Drawing for the job (mm, zero at the part's lowest x, y, z). A direction names the side the tool comes from. Round coordinates to 2 decimals unless told otherwise and drop trailing zeros. Loops run counter-clockwise (first coordinate to the right, second up) from the corner with the lowest first, then second, coordinate; pieces in that order, holes last. Notation, with made-up numbers: M 27,-22.5 L 74,-22.5 A13 ccw 74,-17.5 Z; hole C -13,81.5 d6. An arc over 180 degrees is marked long. Use a Markdown table: item, result. Add a question column.
Q1. Tool access for the marked faces 1, 2, 3, 4 and 5: list every direction of +Z, -Z, +X, -X, +Y, -Y with a clear straight run to the whole face (end or side of a thin tool).
Q2. Probe line 1 (X direction, y = 51.3, z = 29.2); line 2 (Y direction, x = 5, z = 28.85); line 3 (X direction, y = 2, z = 29). List the from-to ranges inside material, lowest first. Write a range as from..to.
Q3. Cut at C-C (x = 10). Give the cut face in (y, z).
Q4. Cut at A-A (y = 2.7). Give the cut face in (x, z), plus the area to 3 significant figures.
Q5. Cut at D-D (z = 9.5). Give the cut face in (x, y).
Q6. Cut at B-B (x = 5). Give the cut face in (y, z).
Q7. Pin check, flat tips, straight feed: pin 1 (3.5 mm diameter, centred on x = 13.5, y = 49, fed in from +Z); pin 2 (6.5 mm diameter, centred on x = 14.9, y = 2.7, fed in from -Z); pin 3 (3 mm diameter, centred on x = 5, z = 32, fed in from -Y); pin 4 (4 mm diameter, centred on x = 5, y = 51.3, fed in from -Z). Stop position of each tip, or through.
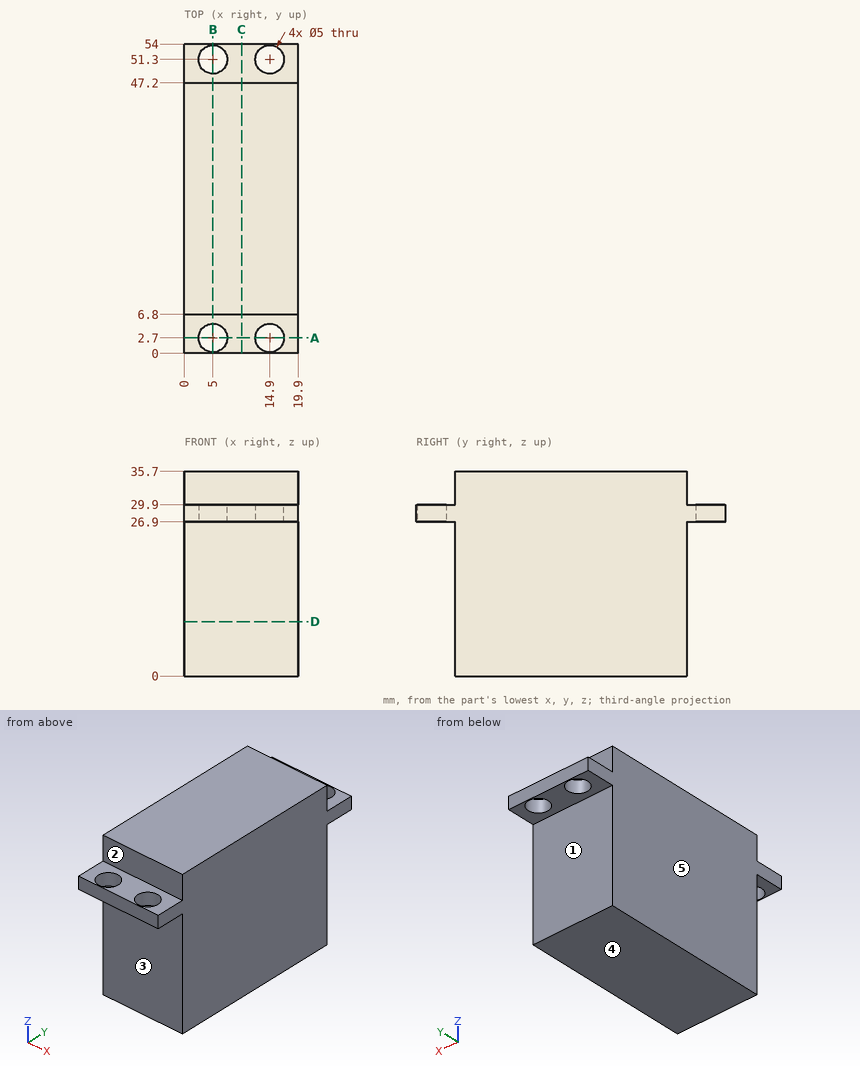
Checked values:
| question | item | result |
|---|---|---|
| 1 | face 1 | -Z, +X, -X, +Y |
| 1 | face 2 | +Z, +X, -X, -Y |
| 1 | face 3 | -Z, +X, -X, -Y |
| 1 | face 4 | -Z, +X, -X, +Y, -Y |
| 1 | face 5 | +Z, -Z, -X, +Y, -Y |
| 2 | line 1 | x = 0..2.5, 7.5..12.4, 17.4..19.9 |
| 2 | line 2 | y = 0..0.2, 5.2..48.8, 53.8..54 |
| 2 | line 3 | x = 0..2.6, 7.4..12.5, 17.3..19.9 |
| 3 | outline | M 0,26.9 L 6.8,26.9 L 6.8,0 L 47.2,0 L 47.2,26.9 L 54,26.9 L 54,29.9 L 47.2,29.9 L 47.2,35.7 L 6.8,35.7 L 6.8,29.9 L 0,29.9 Z |
| 4 | outline | M 0,26.9 L 2.5,26.9 L 2.5,29.9 L 0,29.9 Z; M 7.5,26.9 L 12.4,26.9 L 12.4,29.9 L 7.5,29.9 Z; M 17.4,26.9 L 19.9,26.9 L 19.9,29.9 L 17.4,29.9 Z |
| 4 | area | 29.7 mm^2 |
| 5 | outline | M 0,6.8 L 19.9,6.8 L 19.9,47.2 L 0,47.2 Z |
| 6 | outline | M 0,26.9 L 0.2,26.9 L 0.2,29.9 L 0,29.9 Z; M 5.2,26.9 L 6.8,26.9 L 6.8,0 L 47.2,0 L 47.2,26.9 L 48.8,26.9 L 48.8,29.9 L 47.2,29.9 L 47.2,35.7 L 6.8,35.7 L 6.8,29.9 L 5.2,29.9 Z; M 53.8,26.9 L 54,26.9 L 54,29.9 L 53.8,29.9 Z |
| 7 | pin 1 | stops at z = 29.9 |
| 7 | pin 2 | stops at z = 26.9 |
| 7 | pin 3 | stops at y = 6.8 |
| 7 | pin 4 | passes through |
